The listing builds one solid part. Answer for the finished solid, in the listing's coordinates (mm). A direction names the side the tool comes from. Coordinates: 2 decimals unless noted, no trailing zeros. Order: outer loops, then holes, each group sorted by start corner. A loop starts at its lowest first (then second) coordinate and runs counter-clockwise, first axis right, second up. Notation, with made-up numbers: (60.25, 83) -> (89.25, 83) arc R14 cw to (89.25, 110) -> close; hole circle Ø4 at (44, 33.5). An arc over 180 degrees is marked (long way). Write each question's results on one line, items separated by ' | '. Start each with the question number.
(1) The part is cut by section C-C, the plane x = 0.5. Give the vertices of the cut face in (y, z), then the cut area to 3 significant figures.
(2) A tool of negligible diameter and unlimited length cuts with its end or side. For faces 1 (the face through (2, -150, -2)), 2 (the face through (-1.08, -73.95, -4.88)), 3 (the face through (-0.54, 2.46, -2.44)), from which of +Z, -Z, +X, -X, +Y, -Y can it reach the whole face along a straight path? Write none if from no direction.
(3) The part is cut by section A-A, the plane z = 0. Give the vertices of the cut face in (x, y).
(4) The part is cut by section B-B, the plane y = -55. Give the vertices of the cut face in (x, z), then the cut area to 3 significant figures.
(5) Straight lines are drawn through the part: L1, parallel to Z at x = -0.5, y = -7.5; L2, parallel to Y at x = -4.25, z = 1.25; L3, parallel to X at y = -80.5, z = -0.25. For each, find the intervals that lie inside material, in ascending order.
(6) Given pin 1 (4 mm diameter, centred on x = -3, y = -137.5, fed in from -Z); pin 2 (5 mm diameter, centred on y = -117, z = 3, fed in from -X), each flat-ended and moving along its own axis, determine where each tip first touches the part or whether it passes through.
```python
from build123d import *

# Parameters (mm, degrees)
F0_R     = 5
F1_DEPTH = 150
F2_R     = 2.5
F3_DEPTH = 5
F4_R     = 2.5
F5_DEPTH = 155


with BuildPart() as f1:
    # F0 (on Front) → F1 (new body)
    with BuildSketch(Plane.XZ):
        Circle(F0_R)
    extrude(amount=F1_DEPTH)

    # F2 (on Front) → F3 (join)
    with BuildSketch(Plane.XZ):
        Circle(F2_R)
    extrude(amount=-F3_DEPTH)

    # F4 (on Front) → F5 (join)
    with BuildSketch(Plane.XZ):
        Circle(F4_R)
    extrude(amount=F5_DEPTH)


solid = f1.part
```
Established:
1) outline: (-155, -2.45) -> (-150, -2.45) -> (-150, -4.97) -> (0, -4.97) -> (0, -2.45) -> (5, -2.45) -> (5, 2.45) -> (0, 2.45) -> (0, 4.97) -> (-150, 4.97) -> (-150, 2.45) -> (-155, 2.45) -> close | area: 1,540 mm^2
2) face 1: -Y | face 2: +Y, -Y | face 3: +Y
3) outline: (-5, -150) -> (-2.5, -150) -> (-2.5, -155) -> (2.5, -155) -> (2.5, -150) -> (5, -150) -> (5, 0) -> (2.5, 0) -> (2.5, 5) -> (-2.5, 5) -> (-2.5, 0) -> (-5, 0) -> close
4) outline: circle Ø10 at (0, 0) | area: 78.5 mm^2
5) L1: z = -4.97 to 4.97 | L2: y = -150 to 0 | L3: x = -4.99 to 4.99
6) pin 1: stops at z = -4.9 | pin 2: stops at x = -4.97
